The figure shows three views and two pictorial views of one solid part (mm, origin at its lowest corner). Answer the questions. A direction names the side the tool comes from. Round coordinates to 2 decimals unless told otherwise and drop trailing zeros. Write each loop counter-clockwise with the first axis right and the second up, starting at its lowest first coordinate (ties: lowest second). Pieces come first, ordered by that corner, then holes. Notation, with made-up numbers: (50, 35) -> (66, 35) arc R26 cw to (66, 68) -> close; hole circle Ø6 at (-15.5, 31). An arc over 180 degrees is marked (long way). One line per item, written item: value.
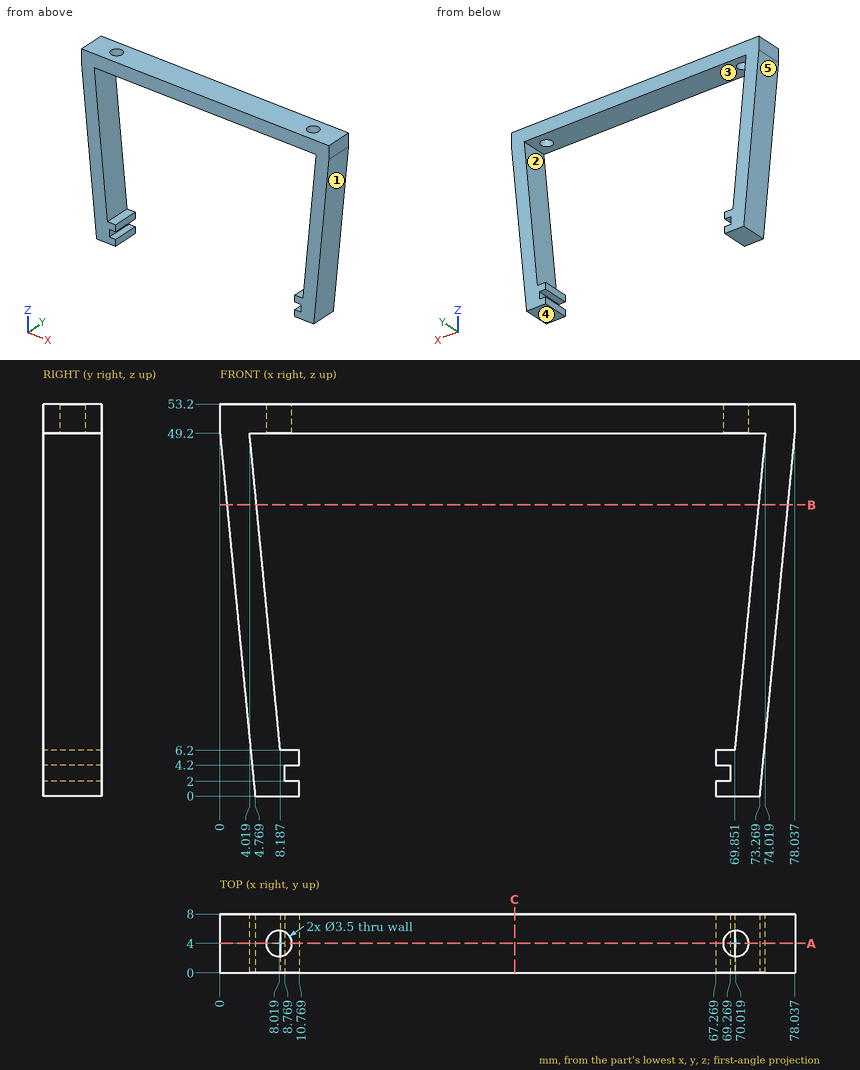
(1) Find section A-A on y = 4. Give the number of separate pieces and of enclosed holes in the cut face, plus the area to 3 significant figures.
Reported:
separate pieces: 3
enclosed holes: 0
area: 699 mm2
(2) A tool of negligible diameter and unlimited length cuts with its end or side. For the marked faces 1 and 2, from which of +Z, -Z, +X, -X, +Y, -Y can it reach the whole face along a straight path? Write none if from no direction.
Reported:
face 1: -Z, +X, +Y, -Y
face 2: +Y, -Y
(3) Flat-ended cylindrical pins translate along their axes: pin 1 Ø2 at (y, z) = (4, 4.5) entering from -X (1 decimal); pin 2 Ø3 at (y, z) = (4.5, 18.5) entering from -X; pin 3 Ø1.8 at (y, z) = (3, 2.5) entering from +X. Find the tip coordinate at first contact, or state that the pin passes through.
Reported:
pin 1: stops at x = 4.2
pin 2: stops at x = 2.83
pin 3: stops at x = 73.6
(4) For a pull along X with two mould halves and no side action, classify the marked faces 3, 4 and 5 as pulls with the +X half, pulls with the -X half, needs draft (parallel to the pull), parting line crosses it, or undercut.
Reported:
face 3: undercut
face 4: needs draft
face 5: pulls with the -X half
(5) Consider probe 1 along Z at (x, y) = (32, 7.5); probe 2 along X at (y, z) = (7.5, 48) (1 decimal); probe 3 along X at (y, z) = (3, 7.5) (1 decimal). Determine where each line is inside the solid, lowest interval first.
Reported:
probe 1: z = 49.2 to 53.2
probe 2: x = 0.1 to 4.1, 73.9 to 77.9
probe 3: x = 4 to 8.1, 70 to 74
(6) Find section C-C on x = 40. Give the vertices of the cut face in (y, z), plus the area to 3 significant figures.
Reported:
outline: (0, 49.2) -> (8, 49.2) -> (8, 53.2) -> (0, 53.2) -> close
area: 32.0 mm2
(7) Find section B-B on z = 39.5. Give the vertices of the cut face in (x, y), plus the area to 3 significant figures.
Reported:
outline: (0.94, 0) -> (4.96, 0) -> (4.96, 8) -> (0.94, 8) -> close; (73.08, 0) -> (77.1, 0) -> (77.1, 8) -> (73.08, 8) -> close
area: 64.3 mm2
